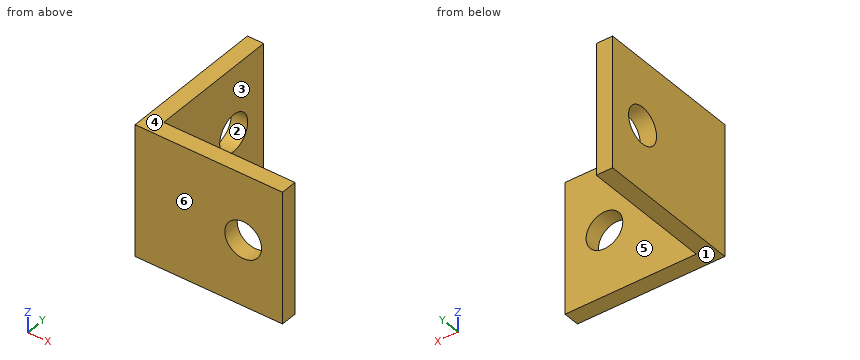
from build123d import *

# Parameters (mm, degrees)
EXTRUDE1_DEPTH     = 12.7
SKETCH2_R          = 1.778
CUT_EXTRUDE1_DEPTH = 7.1374
SKETCH4_R          = 1.778
CUT_EXTRUDE2_DEPTH = 7.1374


with BuildPart() as part:
    # Sketch1 → Extrude1 (new body)
    with BuildSketch(Plane.XY):
        Polygon((0, 0), (-14.2748, 0), (-14.2748, 14.2748), (-12.7, 14.2748), (-12.7, 1.5748), (0, 1.5748), align=None)
    extrude(amount=EXTRUDE1_DEPTH)

    # Sketch2 → Cut-Extrude1 (cut)
    with BuildSketch(Plane(origin=(-12.7, 0, 0), x_dir=(0, 0, -1), z_dir=(1, 0, 0))):
        with Locations((-6.35, 10.4648)):
            Circle(SKETCH2_R)
    extrude(amount=-CUT_EXTRUDE1_DEPTH, mode=Mode.SUBTRACT)

    # Sketch4 → Cut-Extrude2 (cut)
    with BuildSketch(Plane(origin=(0, 1.5748, 0), x_dir=(-1, 0, 0), z_dir=(0, 1, 0))):
        with Locations((3.81, 6.35)):
            Circle(SKETCH4_R)
    extrude(amount=-CUT_EXTRUDE2_DEPTH, mode=Mode.SUBTRACT)


solid = part.part
Part model, mm, in its own coordinate system. Face numbers are marked on the shaded views. A direction names the side the tool comes from. Give positions to 0.01 mm unless a question says otherwise; leave off trailing zeros. Loops run counter-clockwise (first coordinate to the right, second up) from the corner with the lowest first, then second, coordinate; pieces in that order, holes last. Notation, with made-up numbers: (-17, 5) -> (15, 5) arc R12 ccw to (15, 15) -> close; hole circle Ø1 at (-32, 66.25). An arc over 180 degrees is marked (long way). Write each question's results on one line, items separated by ' | '. Start each with the question number.
Q1. Band-saw the part on C-C on y = 1. List the corners of the cut face in (x, z), plus the area to 3 significant figures.
Q2. Pin check, flat tips, straight feed: P1, Ø5.5, axis at x = -3.81, z = 6.35, coming from the -Y side; P2, Ø4, axis at y = 9, z = 3.5, coming from the +X side; P3, Ø6, axis at x = -9.5, z = 2, coming from the +Y side. Stop position of each tip, or through.
Q3. Which spindle directions (+Z, -Z, +X, -X, +Y, -Y) get a long thin tool onto all of the face, cutting with end or side? Do the marked faces 5 and 6. Say none if no direction does.
Q4. Band-saw the part on A-A on x = -3.81. List the corners of the cut face in (y, z), plus the area to 3 significant figures.
Q5. Band-saw the part on B-B on z = 6.35. List the corners of the cut face in (x, y), plus the area to 3 significant figures.
Q6. Wall check: L1, parallel to Y at x = -13.65, z = 6.35; L2, parallel to X at y = 6.75, z = 9.5; L3, parallel to Y at x = -10.25, z = 4.75. Give the ranges that are in metal, low to high.
Q7. Pull direction Z, two halves, no side cores. Call the marked faces 1, 2, 3 and 4: +Z half, -Z half, draft (parallel to the pull), parting line (faces both ways), or undercut.
Q8. Band-saw the part on D-D on y = 11.5. List the corners of the cut face in (x, z).
Results are:
1) outline: (-14.27, 0) -> (0, 0) -> (0, 12.7) -> (-14.27, 12.7) -> close; hole circle Ø3.56 at (-3.81, 6.35) | area: 171 mm²
2) P1: stops at y = 0 | P2: stops at x = -12.7 | P3: stops at y = 1.57
3) face 5: +Z, -Z, +X, +Y | face 6: +Z, -Z, +X, -X, -Y
4) outline: (0, 0) -> (1.57, 0) -> (1.57, 4.57) -> (0, 4.57) -> close; (0, 8.13) -> (1.57, 8.13) -> (1.57, 12.7) -> (0, 12.7) -> close | area: 14.4 mm²
5) outline: (-14.27, 0) -> (-5.59, 0) -> (-5.59, 1.57) -> (-12.7, 1.57) -> (-12.7, 8.69) -> (-14.27, 8.69) -> close; (-14.27, 12.24) -> (-12.7, 12.24) -> (-12.7, 14.27) -> (-14.27, 14.27) -> close; (-2.03, 0) -> (0, 0) -> (0, 1.57) -> (-2.03, 1.57) -> close | area: 31.3 mm²
6) L1: y = 0 to 8.69, 12.24 to 14.27 | L2: x = -14.27 to -12.7 | L3: y = 0 to 1.57
7) face 1: -Z half | face 2: undercut | face 3: draft | face 4: +Z half
8) outline: (-14.27, 0) -> (-12.7, 0) -> (-12.7, 4.9) -> (-14.27, 4.9) -> close; (-14.27, 7.8) -> (-12.7, 7.8) -> (-12.7, 12.7) -> (-14.27, 12.7) -> close
